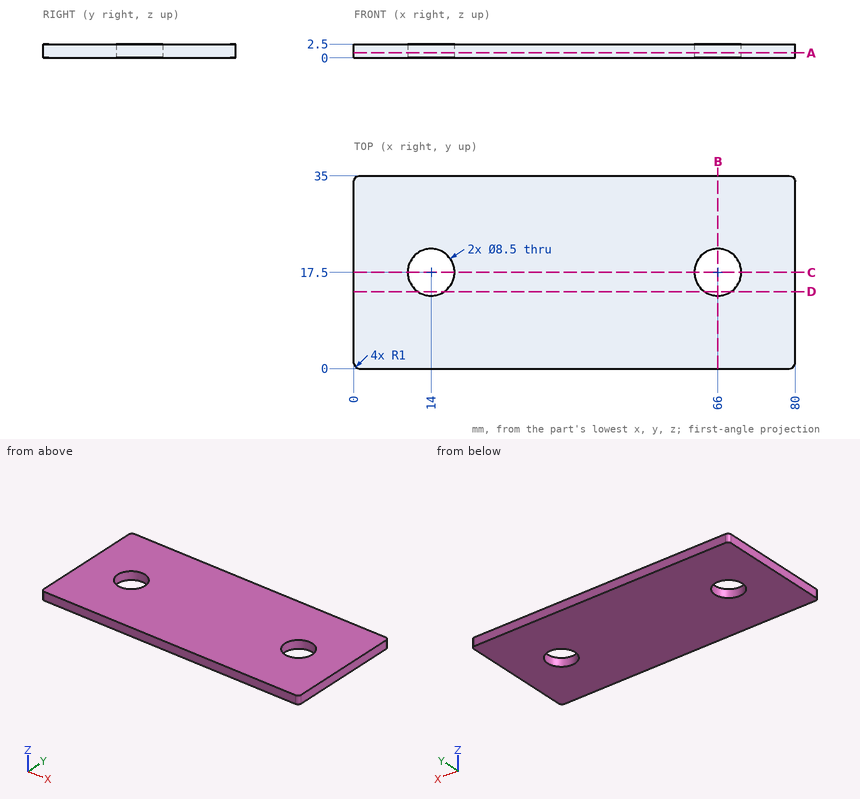
Print and shaded views of the part. All mm, measured from the part's lowest x, y and z. Give positions to 0.01 mm unless a question says otherwise; leave off trailing zeros. Loops run counter-clockwise (first coordinate to the right, second up) from the corner with the lowest first, then second, coordinate; pieces in that order, holes last.
1) Saw through at D-D (y = 14). Write the cut outline in (x, z).
2) Saw through at B-B (x = 66). Write the cut outline in (y, z), plus the area to 4 significant figures.
3) Saw through at A-A (z = 0.9). Write the cut outline in (x, y).
4) Wall check: line 1 (X direction, y = 14, z = 2.05); line 2 (X direction, y = 17, z = 0.65); line 3 (Y direction, x = 66, z = 1.2). Give the ranges that are in metal, low to high.
5) Saw through at C-C (y = 17.5). Write the cut outline in (x, z), plus the area to 4 significant figures.
Answer block:
1. outline: (0, 0) - (11.59, 0) - (11.59, 2.5) - (0, 2.5) - close; (16.41, 0) - (63.59, 0) - (63.59, 2.5) - (16.41, 2.5) - close; (68.41, 0) - (80, 0) - (80, 2.5) - (68.41, 2.5) - close
2. outline: (0, 0) - (13.25, 0) - (13.25, 2.5) - (0, 2.5) - close; (21.75, 0) - (35, 0) - (35, 2.5) - (21.75, 2.5) - close
2. area: 66.25 mm2
3. outline: (0, 1) arc R1 ccw to (1, 0) - (79, 0) arc R1 ccw to (80, 1) - (80, 34) arc R1 ccw to (79, 35) - (1, 35) arc R1 ccw to (0, 34) - close; hole circle Ø8.5 at (14, 17.5); hole circle Ø8.5 at (66, 17.5)
4. line 1: x = 0 to 11.59, 16.41 to 63.59, 68.41 to 80
4. line 2: x = 0 to 9.78, 18.22 to 61.78, 70.22 to 80
4. line 3: y = 0 to 13.25, 21.75 to 35
5. outline: (0, 0) - (9.75, 0) - (9.75, 2.5) - (0, 2.5) - close; (18.25, 0) - (61.75, 0) - (61.75, 2.5) - (18.25, 2.5) - close; (70.25, 0) - (80, 0) - (80, 2.5) - (70.25, 2.5) - close
5. area: 157.5 mm2
